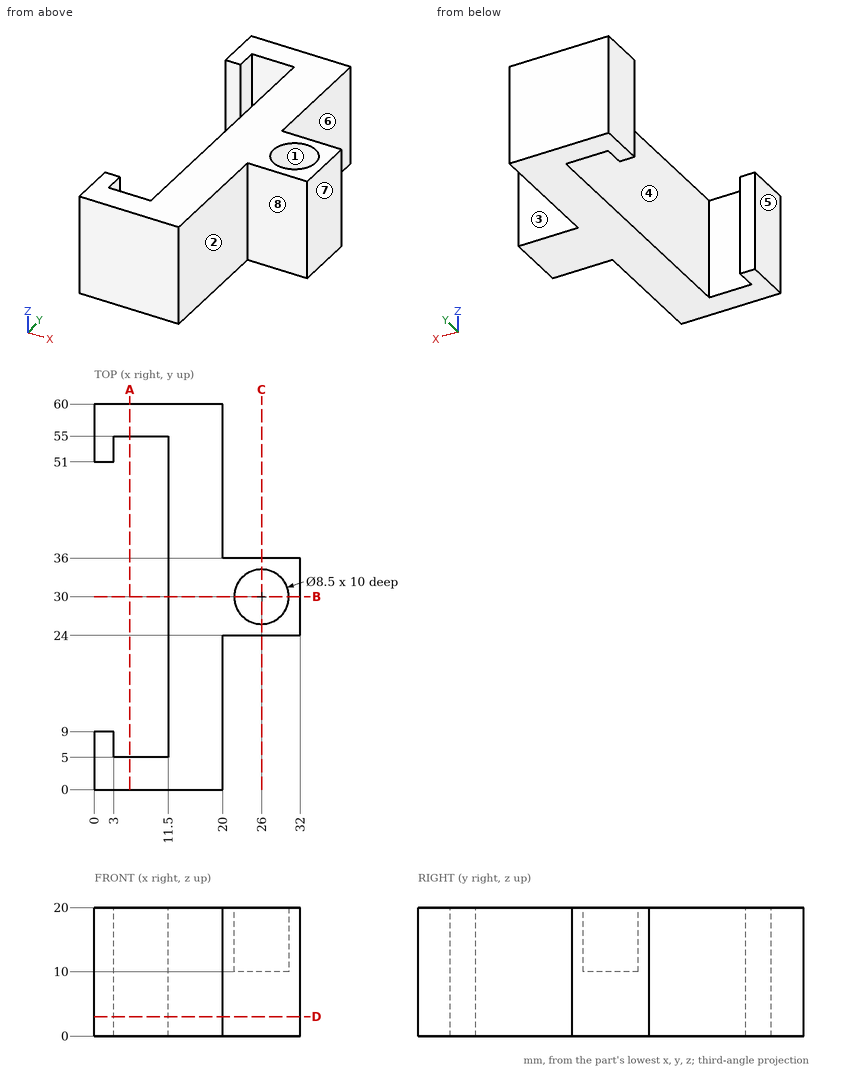
Design review of the part shown in the three views and the two pictorial views. Dimensions are in mm from the part's minimum x, y and z. A direction names the side the tool comes from. Round coordinates to 2 decimals unless told otherwise and drop trailing zeros. Order: outer loops, then holes, each group sorted by start corner. A loop starts at its lowest first (then second) coordinate and runs counter-clockwise, first axis right, second up.
Item 1: Add section B-B, the plane y = 30. State the section outline as (x, z) points, and give its area (3 significant figures).
Working result:
outline: (11.5, 0) - (32, 0) - (32, 20) - (30.25, 20) - (30.25, 10) - (21.75, 10) - (21.75, 20) - (11.5, 20) - close
area: 325 mm2
Item 2: Add section C-C, the plane x = 26. State the section outline as (y, z) points.
Working result:
outline: (24, 0) - (36, 0) - (36, 20) - (34.25, 20) - (34.25, 10) - (25.75, 10) - (25.75, 20) - (24, 20) - close
Item 3: Machinability: for the marked faces 4, 5, 6, 7 and 8, which of the approach directions +Z, -Z, +X, -X, +Y, -Y give a long, thin tool a straight path to every point of the face, cutting with its end or side? Answer none if there is none.
Working result:
face 4: +Z, -Z
face 5: +Z, -Z, -X, +Y, -Y
face 6: +Z, -Z, +X, +Y
face 7: +Z, -Z, +X, +Y, -Y
face 8: +Z, -Z, +X, -Y
Item 4: Draft analysis for pull direction Y (two halves, no side actions). For the marked faces 1, 2 and 3, state which applies: released by +Y, released by -Y, zero draft, split by the parting line, or undercut.
Working result:
face 1: undercut
face 2: zero draft
face 3: released by +Y
Item 5: To check wall thickness, follow probe 1 along Y at (x, z) = (26, 15); probe 2 along X at (y, z) = (54, 1.5); probe 3 along Y at (x, z) = (2.5, 9.25). State the ranges of each line that lie inside material, in increasing order.
Working result:
probe 1: y = 24 to 25.75, 34.25 to 36
probe 2: x = 0 to 3, 11.5 to 20
probe 3: y = 0 to 9, 51 to 60
Item 6: For pin 1 (10 mm diameter, centred on y = 13, z = 2, fed in from +X); pin 2 (6 mm diameter, centred on x = 27, z = 10, fed in from +Y); pin 3 (5 mm diameter, centred on x = 26, y = 30, fed in from +Z), all flat-tipped, find the tip position at first contact; note any pin that passes through.
Working result:
pin 1: stops at x = 20
pin 2: stops at y = 36
pin 3: stops at z = 10
Item 7: Add section D-D, the plane z = 3. State the section outline as (x, y) points, and give its area (3 significant figures).
Working result:
outline: (0, 0) - (20, 0) - (20, 24) - (32, 24) - (32, 36) - (20, 36) - (20, 60) - (0, 60) - (0, 51) - (3, 51) - (3, 55) - (11.5, 55) - (11.5, 5) - (3, 5) - (3, 9) - (0, 9) - close
area: 793 mm2
Item 8: Add section A-A, the plane x = 5.5. State the section outline as (y, z) points, and give its area (3 significant figures).
Working result:
outline: (0, 0) - (5, 0) - (5, 20) - (0, 20) - close; (55, 0) - (60, 0) - (60, 20) - (55, 20) - close
area: 200 mm2
